Geometry check sheet. Reference: the model listing, model coordinates, mm. A direction names the side the tool comes from. Give positions to 0.01 mm unless a question says otherwise; leave off trailing zeros. Order: outer loops, then holes, each group sorted by start corner. A loop starts at its lowest first (then second) coordinate and runs counter-clockwise, first axis right, second up. Notation, with made-up numbers: M 20.25,59.25 L 60.25,59.25 A30 cw 60.25,88.25 Z; hole C 15,59.25 d4. An arc over 180 degrees is marked long. Answer as CSV lines item,"result". Start each with the question number.
Q1. Set-up check for faces 1 (the cylindrical face through (-114.19, 5.03, 83.71)), 2 (the cylindrical face through (-110.86, -85.01, 83.17)): record each of +Z, -Z, +X, -X, +Y, -Y from which the full face is reachable in a straight line by a thin tool's end or side.
Q2. Section check A-A, the plane x = 0. Record the boundary of the cut face in (y, z).
Q3. Go/stop test with flat-tipped pins: pin 1 (6 mm diameter, centred on x = 10.5, z = 124, fed in from -Y); pin 2 (10 mm diameter, centred on x = 48.5, z = 40.5, fed in from -Y); pin 3 (6 mm diameter, centred on y = 110, z = 86, fed in from +X). Record where each tip stops, or that it passes through.
Q4. Section check C-C, the plane z = 111. Record the boundary of the cut face in (x, y), then the cut area to 3 significant figures.
Q5. Thickness scan on line 1 (Y direction, x = 0, z = 125); line 2 (X direction, y = -3, z = 111); line 3 (Y direction, x = -72, z = 120). Record the ranges inside material, lowest first.
Q6. Mould release check, pull along Z, two halves, no side actions. Record for faces 3 (the cylindrical face through (151.42, 47.68, 11.59)), 4 (the flat face through (38, 108, 0)), 5 (the flat face through (34, -150, 25.4)): +Z half, -Z half, draft (parallel to the pull), parting line (faces both ways), or undercut.
```python
from build123d import *

# Parameters (mm, degrees)
F2_R     = 12.7
F3_R     = 2.54
F4_R     = 114.3
F5_DEPTH = 165.101


with BuildPart() as f1:
    # F0 (on Front) → F1 (revolve)
    with BuildSketch(Plane.XZ):
        Polygon((0, 165.1), (0, 0), (158.75, 0), (158.75, 25.4), (139.7, 25.4), (139.7, 139.7), (158.75, 139.7), (158.75, 165.1), align=None)
    revolve(axis=Axis((0, 0, 82.55), (0, 0, 1)))

    # F2
    f2_edges = [f1.edges().sort_by_distance(p)[0] for p in [
        (-139.7, 0, 139.7),
        (-139.7, 0, 25.4),
    ]]
    fillet(f2_edges, radius=F2_R)

    # F3
    f3_edges = [f1.edges().sort_by_distance(p)[0] for p in [
        (-158.75, 0, 25.4),
        (-158.75, 0, 139.7),
    ]]
    fillet(f3_edges, radius=F3_R)

    # F4 (on face) → F5 (cut, through all)
    with BuildSketch(Plane.XY.offset(165.1)):
        Circle(F4_R)
    extrude(amount=-F5_DEPTH, mode=Mode.SUBTRACT)


solid = f1.part
```
Answer block:
1,face 1,"+Z, -Z"
1,face 2,"none"
2,outline,"M -158.75,0 L -114.3,0 L -114.3,165.1 L -158.75,165.1 L -158.75,142.24 A2.54 ccw -156.21,139.7 L -152.4,139.7 A12.7 cw -139.7,127 L -139.7,38.1 A12.7 cw -152.4,25.4 L -156.21,25.4 A2.54 ccw -158.75,22.86 Z; M 114.3,0 L 158.75,0 L 158.75,22.86 A2.54 ccw 156.21,25.4 L 152.4,25.4 A12.7 cw 139.7,38.1 L 139.7,127 A12.7 cw 152.4,139.7 L 156.21,139.7 A2.54 ccw 158.75,142.24 L 158.75,165.1 L 114.3,165.1 Z"
3,pin 1,"stops at y = -139.5"
3,pin 2,"stops at y = -132.75"
3,pin 3,"stops at x = 89.82"
4,outline,"C 0,0 d279.4; hole C 0,0 d228.6"
4,area,"20,300 mm2"
5,line 1,"y = -139.7 to -114.3, 114.3 to 139.7"
5,line 2,"x = -139.67 to -114.26, 114.26 to 139.67"
5,line 3,"y = -119.72 to -88.77, 88.77 to 119.72"
6,face 3,"draft"
6,face 4,"-Z half"
6,face 5,"undercut"
